The figure shows three views and two pictorial views of one solid part (mm, origin at its lowest corner). Answer the questions. Coordinates: 2 decimals unless noted, no trailing zeros. Order: outer loops, then holes, each group sorted by start corner. A loop starts at its lowest first (then second) coordinate and runs counter-clockwise, first axis right, second up. Notation, with made-up numbers: (80, 40.5) -> (121, 40.5) arc R20 ccw to (121, 74.5) -> close; hole circle Ø3 at (-0.75, 7.25). An arc over 180 degrees is marked (long way). Write item = value, one per line. Start each with the question number.
Q1. Flat-ended cylindrical pins translate along their axes: pin 1 (0.8 mm diameter, centred on x = 46, y = 1.5, fed in from +Z); pin 2 (0.9 mm diameter, centred on x = 1.5, y = 1, fed in from -Z); pin 3 (1.5 mm diameter, centred on y = 2, z = 57, fed in from -X). Find the tip coordinate at first contact, or state that the pin passes through.
Q2. Straight lines are drawn through the part: L1, parallel to Z at x = 1.35, y = 2.4 (1 decimal); L2, parallel to X at y = 2.35, z = 53 (1 decimal); L3, parallel to Z at x = 86.5, y = 2.8. For each, find the intervals that lie inside material, in ascending order. Write a range as from..to.
Q3. The part is cut by section B-B, the plane z = 37. Determine the outline of the cut face in (x, y).
Q4. The part is cut by section C-C, the plane x = 87. Determine the outline of the cut face in (y, z), plus the area to 3 significant figures.
Q5. The part is cut by section A-A, the plane x = 1.35. Determine the outline of the cut face in (y, z) (1 decimal).
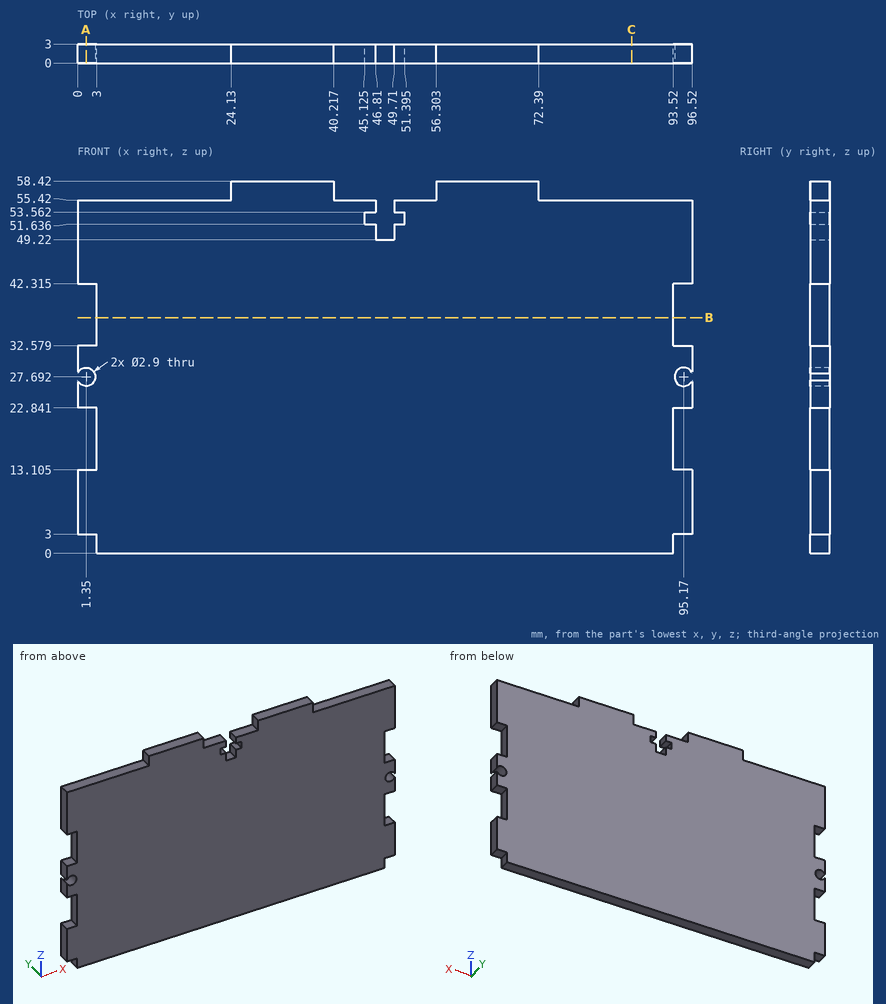
Model answer:
q1.pin_1 = 55.42
q1.pin_2 = 3
q1.pin_3 = 24.13
q2.L1 = 3..13.1, 22.8..26.2, 29.1..32.6, 42.3..55.4
q2.L2 = 0..45.1, 51.4..96.5
q2.L3 = 0..55.42
q3.outline = (3, 0) -> (93.52, 0) -> (93.52, 3) -> (3, 3) -> close
q4.outline = (0, 0) -> (3, 0) -> (3, 55.42) -> (0, 55.42) -> close
q4.area = 166 mm2
q5.outline = (0, 3) -> (3, 3) -> (3, 13.1) -> (0, 13.1) -> close; (0, 22.8) -> (3, 22.8) -> (3, 26.2) -> (0, 26.2) -> close; (0, 29.1) -> (3, 29.1) -> (3, 32.6) -> (0, 32.6) -> close; (0, 42.3) -> (3, 42.3) -> (3, 55.4) -> (0, 55.4) -> close
